from build123d import *

# Parameters (mm, degrees)
SKETCH_1_R          = 40
EXTRUDE_1_DEPTH     = 2
SKETCH_2_R          = 34
EXTRUDE_2_DEPTH     = 6
SKETCH_3_R          = 27.5
CUT_EXTRUDE_1_DEPTH = 57.885850613
SKETCH_4_W          = 46.937334883
SKETCH_4_H          = 4
CUT_EXTRUDE_2_DEPTH = 2


with BuildPart() as part:
    # 草图1 → 凸台-拉伸1 (new body)
    with BuildSketch(Plane.XY):
        Circle(SKETCH_1_R)
    extrude(amount=EXTRUDE_1_DEPTH)

    # 草图2 → 凸台-拉伸2 (add)
    with BuildSketch(Plane.XY):
        Circle(SKETCH_2_R)
    extrude(amount=EXTRUDE_2_DEPTH)

    # 草图3 → 切除-拉伸1 (cut, through all)
    with BuildSketch(Plane.XY.offset(6)):
        Circle(SKETCH_3_R)
    extrude(amount=-CUT_EXTRUDE_1_DEPTH, mode=Mode.SUBTRACT)

    # 草图4 → 切除-拉伸2 (cut)
    with BuildSketch(Plane.XY.offset(6)):
        with Locations((30.403538279, 0)):
            Rectangle(SKETCH_4_W, SKETCH_4_H)
    extrude(amount=-CUT_EXTRUDE_2_DEPTH, mode=Mode.SUBTRACT)


solid = part.part
CAD build for the part. Positions are in the model's coordinates, mm. A direction names the side the tool comes from. Coordinates: 2 decimals unless noted, no trailing zeros. Write each loop counter-clockwise with the first axis right and the second up, starting at its lowest first coordinate (ties: lowest second). Pieces come first, ordered by that corner, then holes. Notation, with made-up numbers: M -36,63 L 19,63 A14 ccw 19,71 Z; hole C -25.5,21.5 d7. An arc over 180 degrees is marked long. Return JSON: item names as keys, results as strings.
Item 1: Slice it at A-A, the plane x = 0. Write the cut outline in (y, z), and give its area (3 significant figures).
Findings below:
{"outline": "M -40,0 L -27.5,0 L -27.5,6 L -34,6 L -34,2 L -40,2 Z; M 27.5,0 L 40,0 L 40,2 L 34,2 L 34,6 L 27.5,6 Z", "area": "102 mm2"}
Item 2: Slice it at C-C, the plane y = -31. Write the cut outline in (x, z).
Findings below:
{"outline": "M -25.28,0 L 25.28,0 L 25.28,2 L 13.96,2 L 13.96,6 L -13.96,6 L -13.96,2 L -25.28,2 Z"}
Item 3: Probe line 1 (Y direction, x = 0, z = 3.95); line 2 (Y direction, x = 0, z = 1.95). List the from-to ranges inside material, lowest first. Write a range as from..to.
Findings below:
{"line 1": "y = -34..-27.5, 27.5..34", "line 2": "y = -40..-27.5, 27.5..40"}
Item 4: Two-plate mould, pull along Y, no slides. Class faces 1 (the cylindrical face through (-8.67, -39.05, 0.99)), 2 (the flat face through (-3, 28, 6)), 3 (the flat face through (31, 0, 4)): +Y half, -Y half, draft (parallel to the pull), parting line (faces both ways), or undercut.
Findings below:
{"face 1": "parting line", "face 2": "draft", "face 3": "undercut"}
Item 5: Drop flat-ended pins along their axis: pin 1 Ø1.5 at (y, z) = (-20.5, 4.5) entering from +X; pin 2 Ø1 at (x, z) = (31, 5) entering from +Y (3 decimals); pin 3 Ø3 at (x, z) = (19.5, 0.5) entering from +Y. Give the stop position or say it passes through.
Findings below:
{"pin 1": "stops at x = 27.68", "pin 2": "stops at y = 15.025", "pin 3": "stops at y = 35.72"}
Item 6: Slice it at D-D, the plane x = -30. Write the cut outline in (y, z).
Findings below:
{"outline": "M -26.46,0 L 26.46,0 L 26.46,2 L 16,2 L 16,6 L -16,6 L -16,2 L -26.46,2 Z"}
Item 7: Slice it at B-B, the plane y = 0. Write the cut outline in (x, z).
Findings below:
{"outline": "M -40,0 L -27.5,0 L -27.5,6 L -34,6 L -34,2 L -40,2 Z; M 27.5,0 L 40,0 L 40,2 L 34,2 L 34,4 L 27.5,4 Z"}
Item 8: Which spindle directions (+Z, -Z, +X, -X, +Y, -Y) get a long thin tool onto all of the face, cutting with end or side? Do faces 4 (the flat face through (-18, -29.4, 2)), 5 (the flat face through (-9.4, -26.1, 0)), 6 (the flat face through (31, -2, 5)). Say none if no direction does.
Findings below:
{"face 4": "+Z", "face 5": "-Z, +X, -X, +Y, -Y", "face 6": "+Z, +X"}
